Work out the finished part from the listing and answer in its coordinate system (mm). A direction names the side the tool comes from. Round coordinates to 2 decimals unless told otherwise and drop trailing zeros. Order: outer loops, then holes, each group sorted by start corner. A loop starts at its lowest first (then second) coordinate and runs counter-clockwise, first axis right, second up. Notation, with made-up numbers: M 71.5,15 L 125.5,15 A7 cw 125.5,23 Z; hole C -37,-29 d4. An arc over 180 degrees is marked long. Return JSON: item names as keys, results as strings.
from build123d import *

# Parameters (mm, degrees)
F0_R     = 15
F0_R_2   = 5
F0_R_3   = 25
F1_DEPTH = 25


with BuildPart() as f1:
    # F0 (on Top) → F1 (new body)
    with BuildSketch(Plane.XY):
        with BuildLine():
            Line((-54.824, 0), (0, 0))
            Line((0, 0), (54.824, 0))
            Line((54.824, 0), (60, 5.17583))
            Line((60, 5.17583), (60, 20))
            Line((60, 20), (100, 20))
            Line((100, 20), (100, 35))
            Line((100, 35), (100, 95))
            ThreePointArc((100, 95), (92.67767, 112.67767), (75, 120))
            Line((75, 120), (-5, 120))
            Line((-5, 120), (-76, 120))
            Line((-76, 120), (-100, 108))
            Line((-100, 108), (-100, 20))
            Line((-100, 20), (-70, 20))
            Line((-70, 20), (-60, 20))
            Line((-60, 20), (-60, 5.176))
            Line((-60, 5.176), (-54.824, 0))
        make_face()
        with Locations((-70, 50)):
            Circle(F0_R, mode=Mode.SUBTRACT)
        with Locations((80, 35)):
            Circle(F0_R_2, mode=Mode.SUBTRACT)
        with Locations((-5, 90)):
            Circle(F0_R_3, mode=Mode.SUBTRACT)
    extrude(amount=F1_DEPTH)


solid = f1.part
Item 1: Which of the six approach directions +Z, -Z, +X, -X, +Y, -Y give full straight-line access (tool end or side, diameter ignored) to faces 1 (the flat face through (-60, 13, 12)), 2 (the flat face through (60, 12, 12)), 3 (the cylindrical face through (-71.953, 64.872, 12.325))?
Output:
{"face 1": "+Z, -Z, -X, -Y", "face 2": "+Z, -Z, +X, -Y", "face 3": "+Z, -Z"}
Item 2: The mould has two halves that part along X. Classify faces 4 (the flat face through (-1, 61, 25)), 5 (the cylindrical face through (84.77, 36.5, 12.32)), 6 (the flat face through (-88, 114, 12)): pulls with the +X half, pulls with the -X half, needs draft (parallel to the pull), parting line crosses it, or undercut.
Output:
{"face 4": "needs draft", "face 5": "undercut", "face 6": "pulls with the -X half"}
Item 3: Find section B-B (y = 50). Determine the outline of the cut face in (x, z), plus the area to 3 significant figures.
Output:
{"outline": "M -100,0 L -85,0 L -85,25 L -100,25 Z; M -55,0 L 100,0 L 100,25 L -55,25 Z", "area": "4,250 mm^2"}
Item 4: Find section A-A (x = -70). Determine the outline of the cut face in (y, z), plus the area to 3 significant figures.
Output:
{"outline": "M 20,0 L 35,0 L 35,25 L 20,25 Z; M 65,0 L 120,0 L 120,25 L 65,25 Z", "area": "1,750 mm^2"}
Item 5: Each of these flat-tipped pins is pushed along its axis until it touches: pin 1 (12.5 mm diameter, centred on x = 76.5, z = 16.5, fed in from -Y); pin 2 (7.5 mm diameter, centred on y = 11, z = 14.5, fed in from -X). Where does it stop, or does it pass through?
Output:
{"pin 1": "stops at y = 20", "pin 2": "stops at x = -60"}
Item 6: Find section C-C (z = 18). Determine the outline of the cut face in (x, y), plus the area to 3 significant figures.
Output:
{"outline": "M -100,20 L -60,20 L -60,5.18 L -54.82,0 L 54.82,0 L 60,5.18 L 60,20 L 100,20 L 100,95 A25 ccw 75,120 L -76,120 L -100,108 Z; hole C -70,50 d30; hole C -5,90 d50; hole C 80,35 d10", "area": "19,300 mm^2"}
Item 7: Consider line 1 along X through (y, z) = (37, 11); line 2 along Y through (x, z) = (-5, 12.5); line 3 along Y through (x, z) = (12, 3.75). Determine where each line is inside the solid, lowest interval first. Write a range as [from, to].
Output:
{"line 1": "x = [-100, -77.48], [-62.52, 75.42], [84.58, 100]", "line 2": "y = [0, 65], [115, 120]", "line 3": "y = [0, 71.67], [108.33, 120]"}
